Autodesk Inventor part; units mm, degrees
ref_plane "YZ Plane" through (0, 0, 0) normal (1, 0, 0) x (0, 1, 0)
ref_plane "XZ Plane" through (0, 0, 0) normal (0, 1, 0) x (-1, 0, 0)
ref_plane "XY Plane" through (0, 0, 0) normal (0, 0, 1) x (1, 0, 0)
sketch "Sketch1" plane through (0, 0, 0) normal (0, 0, 1) x (1, 0, 0)
  line L0 (-14, 8.7) -> (-14, 6.0607)
  line L1 (-14, 8.7) -> (-14, 6.0607)
  line L2 (-14, 6.0607) -> (-16.5607, 3.5)
  line L3 (-14, 6.0607) -> (-16.5607, 3.5)
  line L4 (-16.5607, 3.5) -> (-18.2, 3.5)
  line L5 (-16.5607, 3.5) -> (-18.2, 3.5)
  line L6 (-18.2, 3.5) -> (-18.2, 6)
  line L7 (-18.2, 3.5) -> (-18.2, 6)
  line L8 (-20, 4.2) -> (-20, 0)
  line L9 (-18.2, 6) -> (-20, 4.2)
  line L10 (-20, 4.2) -> (-20, 0)
  line L11 (-19, -1) -> (-14.8, -1)
  line L12 (-19, -1) -> (-14.8, -1)
  line L13 (-14.8, -1) -> (-13, 0.8)
  line L14 (-14.8, -1) -> (-13, 0.8)
  line L15 (-15.5, 0.8) -> (-15.5, 2.4393)
  line L16 (-13, 0.8) -> (-15.5, 0.8)
  line L17 (-15.5, 0.8) -> (-15.5, 2.4393)
  line L18 (-12.9393, 5) -> (-10.3, 5)
  line L19 (-15.5, 2.4393) -> (-12.9393, 5)
  line L20 (-12.9393, 5) -> (-10.3, 5)
  line L21 (-10, 5.3) -> (-9.7, 5)
  line L22 (-10.3, 5) -> (-10, 5.3)
  line L23 (-13.7, 9) -> (-14, 8.7)
  line L24 (-13.7, 9) -> (-14, 8.7)
  line L25 (-10, 9) -> (-10, 10.0607)
  circle A0 centre (-10, 9) radius 2.5
  arc A1 (-20, 0) -> (-19, -1) centre (-19, 0) ccw
  arc A2 (-20, 0) -> (-19, -1) centre (-19, 0) ccw
  line L26 (-7.0607, 5) -> (-4.5, 2.4393)
  line L27 (-4.5, 2.4393) -> (-4.5, 0.8)
  line L28 (-4.5, 0.8) -> (-7, 0.8)
  line L29 (-7, 0.8) -> (-5.2, -1)
  line L30 (-3.4393, 3.5) -> (-6, 6.0607)
  line L31 (-1.8, 6) -> (-1.8, 3.5)
  line L32 (-1.8, 3.5) -> (-3.4393, 3.5)
  line L33 (0, 4.2) -> (-1.8, 6)
  line L34 (-5.2, -1) -> (-1, -1)
  line L35 (0, 0) -> (0, 4.2)
  arc A3 (-1, -1) -> (0, 0) centre (-1, 0) ccw
  line L36 (-9.7, 5) -> (-7.0607, 5)
  line L37 (-6, 6.0607) -> (-6, 8.7)
  line L38 (-6, 8.7) -> (-6.3, 9)
  line L39 (-10, 5.3) -> (-9.7, 5)
  line L40 (-6, 11.9393) -> (-3.4393, 14.5)
  line L41 (-3.4393, 14.5) -> (-1.8, 14.5)
  line L42 (-1.8, 14.5) -> (-1.8, 12)
  line L43 (-1.8, 12) -> (0, 13.8)
  line L44 (-4.5, 15.5607) -> (-7.0607, 13)
  line L45 (-7, 17.2) -> (-4.5, 17.2)
  line L46 (-4.5, 17.2) -> (-4.5, 15.5607)
  line L47 (-5.2, 19) -> (-7, 17.2)
  line L48 (0, 13.8) -> (0, 18)
  line L49 (-1, 19) -> (-5.2, 19)
  arc A4 (0, 18) -> (-1, 19) centre (-1, 18) ccw
  line L50 (-6, 9.3) -> (-6, 11.9393)
  line L51 (-7.0607, 13) -> (-9.7, 13)
  line L52 (-9.7, 13) -> (-10, 12.7)
  line L53 (-6.3, 9) -> (-6, 9.3)
  line L54 (-12.9393, 13) -> (-15.5, 15.5607)
  line L55 (-15.5, 15.5607) -> (-15.5, 17.2)
  line L56 (-15.5, 17.2) -> (-13, 17.2)
  line L57 (-13, 17.2) -> (-14.8, 19)
  line L58 (-16.5607, 14.5) -> (-14, 11.9393)
  line L59 (-18.2, 12) -> (-18.2, 14.5)
  line L60 (-18.2, 14.5) -> (-16.5607, 14.5)
  line L61 (-20, 13.8) -> (-18.2, 12)
  line L62 (-14.8, 19) -> (-19, 19)
  line L63 (-20, 18) -> (-20, 13.8)
  arc A5 (-19, 19) -> (-20, 18) centre (-19, 18) ccw
  line L64 (-10.3, 13) -> (-12.9393, 13)
  line L65 (-14, 11.9393) -> (-14, 9.3)
  line L66 (-14, 9.3) -> (-13.7, 9)
  line L67 (-10, 12.7) -> (-10.3, 13)
  point P0 (0, 0)
  point P1 (-1, 0)
  point P2 (-1, 18)
  point P3 (-19, 18)
  dimension "d2" = 360
extrude "Extrusion1" add sketch "Sketch1" along normal blind 300
properties part number "20x20x300" material "Aluminum 6061"
The listing builds one solid part. Answer for the finished solid, in the listing's coordinates (mm). Round coordinates to 2 decimals unless told otherwise and drop trailing zeros.
Q1. For a pull along X with two mould halves and no side action, classify faces 1 (the face through (-10.54, 11.44, 147.9)), 2 (the face through (-12, 7, 300)) as released by +X, released by -X, zero draft, split by the parting line, or undercut.
Q2. Find the intervals of material crossed by line 1 (Y direction, x = -10, z = 158); line 2 (Y direction, x = -6.5, z = 225.5); line 3 (X direction, y = 13.5, z = 255.5), in increasing order.
Q3. Given pin 1 Ø0.8 at (x, z) = (-9, 201.5) entering from -Y; pin 2 Ø3 at (y, z) = (11, 226.5) entering from -X; pin 3 Ø1.5 at (y, z) = (7, 133) entering from -X; pin 4 Ø3 at (x, y) = (-10, 9) entering from -Z, each flat-ended and moving along its own axis, determine where each tip first touches the part or whether it passes through.
Completed:
1. face 1: undercut
1. face 2: zero draft
2. line 1: y = 5.3 to 6.5, 11.5 to 12.7
2. line 2: y = 0.3 to 0.8, 4.44 to 13.56, 17.2 to 17.7
2. line 3: x = -19.7 to -18.2, -15.56 to -13.44, -6.56 to -4.44, -1.8 to -0.3
3. pin 1: stops at y = 5
3. pin 2: stops at x = -18.7
3. pin 3: stops at x = -14
3. pin 4: passes through
